Work out the finished part from the listing and answer in its coordinate system (mm). A direction names the side the tool comes from. Coordinates: 2 decimals unless noted, no trailing zeros. Write each loop counter-clockwise with the first axis right and the second up, starting at its lowest first coordinate (ties: lowest second). Pieces come first, ordered by that corner, then holes. Notation, with made-up numbers: (75, -20.5) - (114, -20.5) arc R24 cw to (114, 6.5) - close; hole circle Ø6 at (-20, 52). An arc over 180 degrees is marked (long way). Use one line per item in the form item = value. Start each with the question number.
Item 1: A cutting plane is placed at C-C (z = -62.5). Write down the section's boundary in (x, y), then the cut area to 3 significant figures.
Item 2: A cutting plane is placed at B-B (y = 19). Write down the section's boundary in (x, z), then the cut area to 3 significant figures.
Item 3: Determine the mould class of faces 4 (the flat face through (-0.4, 29, -22.86)), 5 (the cylindrical face through (11.56, 14.37, 15.08)) for opening direction Y: released by +Y, released by -Y, zero draft, split by the parting line, or undercut.
Item 4: Given pin 1 (12 mm diameter, centred on x = 29.5, z = 40.5, fed in from +Y); pin 2 (5.5 mm diameter, centred on x = -54.13, z = 31.25, fed in from -Y); pin 3 (6 mm diameter, centred on x = -6, y = 18, fed in from -Z); pin 4 (2.5 mm diameter, centred on x = 2.5, y = 27.5, fed in from +Z), each flat-ended and moving along its own axis, determine where each tip first touches the part or whether it passes through.
Item 5: A cutting plane is placed at D-D (y = 9.5). Give the number of separate pieces and of enclosed holes in the cut face, then the cut area to 3 significant figures.
Item 6: A cutting plane is placed at A-A (z = 0). Write down the section's boundary in (x, y).
Item 7: Consider probe 1 along Z at (x, y) = (3, 17); probe 2 along Y at (x, z) = (-43, 41); probe 3 along X at (y, z) = (9.5, -61.5). Determine where each line is inside the solid, lowest interval first.
Item 8: For faces 1 (the cylindrical face through (-1.539, 18.73, 34.966)), 2 (the cylindrical face through (0, 6, 59)), 3 (the flat face through (-7, 24, 19)), determine the directions among +Z, -Z, +X, -X, +Y, -Y from which every point of the face is accessible in a straight line to the end or side of a thin tool.
from build123d import *

# Parameters (mm, degrees)
SKETCH3_W         = 41.1
SKETCH3_H         = 5
EXTRUDE2_DEPTH    = 60
SKETCH2_R         = 4.5
EXTRUDE1_DEPTH    = 110.959083299
CIRPATTERN1_COUNT = 6


with BuildPart() as part:
    # Sketch1 → Revolve1 (revolve)
    with BuildSketch(Plane.XY, mode=Mode.PRIVATE) as revolve1_sk:
        Polygon((-10, 0), (-75, 0), (-75, 12), (-35, 12), (-35, 29), (-19, 29), (-19, 5), (-10, 5), align=None)
    revolve(revolve1_sk.sketch.rotate(Axis((0, 0, 0), (0, 1, 0)), 270), axis=Axis((0, 0, 0), (0, 1, 0)))

    # Sketch3 → Extrude2 (cut, symmetric)
    with BuildSketch(Plane(origin=(0, 0, 0), x_dir=(0, 0, -1), z_dir=(1, 0, 0))):
        with Locations((0, 26.5)):
            Rectangle(SKETCH3_W, SKETCH3_H)
    extrude(amount=EXTRUDE2_DEPTH, both=True, mode=Mode.SUBTRACT)

    # Sketch2 → Extrude1 (cut, through all)
    with BuildSketch(Plane.XZ):
        with Locations(Location((-27.5, 0, 0), (0, 0, 270))):
            Circle(SKETCH2_R)
        with Locations(Location((0, -27.5, 0), (0, 0, 270))):
            Circle(SKETCH2_R)
        with Locations(Location((0, 27.5, 0), (0, 0, 270))):
            Circle(SKETCH2_R)
        with Locations(Location((27.5, 0, 0), (0, 0, 270))):
            Circle(SKETCH2_R)
    extrude(amount=-EXTRUDE1_DEPTH, mode=Mode.SUBTRACT)

    # Sketch4 → M8x1.0 Tapped Hole1 (revolve, cut)
    with BuildSketch(Plane(origin=(0, 12, 62.5), x_dir=(0, 0, 1), z_dir=(1, 0, 0))):
        Polygon((0, 0), (0, 23.103012167), (3.5, 21), (3.5, 0), align=None)
    m8x1_0_tapped_hole1 = revolve(axis=Axis((0, 18.35, 62.5), (0, -1, 0)), mode=Mode.SUBTRACT)

    # CirPattern1: M8x1.0 Tapped Hole1 ×6 about axis
    cirpattern1_axis = Axis((0, 0, 0), (0, 1, 0))
    for i in range(1, CIRPATTERN1_COUNT):
        add(m8x1_0_tapped_hole1.rotate(cirpattern1_axis, i * 360 / CIRPATTERN1_COUNT), mode=Mode.SUBTRACT)


solid = part.part
Answer:
q1.outline = (-41.46, 0) - (-3.5, 0) - (-3.5, 12) - (-41.46, 12) - close; (3.5, 0) - (41.46, 0) - (41.46, 12) - (3.5, 12) - close
q1.area = 911 mm²
q2.outline = circle Ø70 at (0, 0); hole circle Ø9 at (-27.5, 0); hole circle Ø38 at (0, 0); hole circle Ø9 at (0, -27.5); hole circle Ø9 at (0, 27.5); hole circle Ø9 at (27.5, 0)
q2.area = 2,460 mm²
q3.face_4 = released by +Y
q3.face_5 = zero draft
q4.pin_1 = 12
q4.pin_2 = through
q4.pin_3 = -34.87
q4.pin_4 = 34.98
q5.separate_pieces = 1
q5.enclosed_holes = 11
q5.area = 16,100 mm²
q6.outline = (-75, 0) - (-32, 0) - (-32, 24) - (-35, 24) - (-35, 12) - (-75, 12) - close; (-23, 0) - (-10, 0) - (-10, 5) - (-19, 5) - (-19, 24) - (-23, 24) - close; (10, 0) - (23, 0) - (23, 24) - (19, 24) - (19, 5) - (10, 5) - close; (32, 0) - (75, 0) - (75, 12) - (35, 12) - (35, 24) - (32, 24) - close
q7.probe_1 = -34.87 to -30.85, -24.15 to -18.76, 18.76 to 24.15, 30.85 to 34.87
q7.probe_2 = 0 to 12
q7.probe_3 = -42.93 to -3.35, 3.35 to 42.93
q8.face_1 = +Y
q8.face_2 = +Y, -Y
q8.face_3 = +X, -X, +Y
